Could you check a few things on this model? Use its own coordinates, in mm. A direction names the side the tool comes from. Coordinates: 2 decimals unless noted, no trailing zeros. Loops run counter-clockwise (first coordinate to the right, second up) from the corner with the lowest first, then second, coordinate; pieces in that order, holes last.
from build123d import *

# Parameters (mm, degrees)
EXTRUDE_1_DEPTH     = 20
CUT_EXTRUDE_1_DEPTH = 2


with BuildPart() as part:
    # 草圖1 → 填料-伸長1 (new body)
    with BuildSketch(Plane.XY):
        with BuildLine():
            Line((-63.421210963, 20), (-60, 20))
            Line((-60, 20), (-60, -20))
            Line((-60, -20), (-63.421210963, -20))
            ThreePointArc((-63.421210963, -20), (0, -66.5), (63.421210963, -20))
            Line((63.421210963, -20), (60, -20))
            Line((60, -20), (60, 20))
            Line((60, 20), (63.421210963, 20))
            ThreePointArc((63.421210963, 20), (0, 66.5), (-63.421210963, 20))
        make_face()
    extrude(amount=EXTRUDE_1_DEPTH)

    # 草圖2 → 除料-伸長1 (cut)
    with BuildSketch(Plane(origin=(0, 0, 0), x_dir=(-1, 0, 0), z_dir=(0, 0, -1))):
        with BuildLine():
            Line((-20, 63.421210963), (-20, -63.421210963))
            ThreePointArc((-20, -63.421210963), (0, -66.5), (20, -63.421210963))
            Line((20, -63.421210963), (20, 63.421210963))
            ThreePointArc((20, 63.421210963), (0, 66.5), (-20, 63.421210963))
        make_face()
    extrude(amount=-CUT_EXTRUDE_1_DEPTH, mode=Mode.SUBTRACT)


solid = part.part
(1) Imagine slicing it at A-A, the plane y = 8.5. Write out the boundary of the cut face in (x, z), and give its area (3 significant figures).
Answers:
outline: (-60, 0) - (-20, 0) - (-20, 2) - (20, 2) - (20, 0) - (60, 0) - (60, 20) - (-60, 20) - close
area: 2,320 mm2
(2) Imagine slicing it at C-C, the plane x = 29.5. Write out the boundary of the cut face in (y, z), and give its area (3 significant figures).
Answers:
outline: (-59.6, 0) - (59.6, 0) - (59.6, 20) - (-59.6, 20) - close
area: 2,380 mm2
(3) We'd pull the mould along Y, two halves only. Please class faces 1 (the face through (62, -20, 10)), 2 (the face through (-37, 1, 0)), 3 (the face through (-1.18, -66.49, 9.86)), 4 (the face through (60, 0, 10)): +Y half, -Y half, draft (parallel to the pull), parting line (faces both ways), or undercut.
Answers:
face 1: undercut
face 2: draft
face 3: -Y half
face 4: undercut
(4) Imagine slicing it at D-D, the plane x = 51.5. Write out the boundary of the cut face in (y, z), and give its area (3 significant figures).
Answers:
outline: (-42.07, 0) - (42.07, 0) - (42.07, 20) - (-42.07, 20) - close
area: 1,680 mm2
(5) I need wall thicknesses on probe 1 along Z at (x, y) = (-18, -40.5); probe 2 along X at (y, z) = (10, 19.25); probe 3 along X at (y, z) = (-47.5, 1). Which ranges of each line are inside material? Lowest first, please.
Answers:
probe 1: z = 2 to 20
probe 2: x = -60 to 60
probe 3: x = -46.54 to -20, 20 to 46.54
(6) Imagine slicing it at B-B, the plane z = 9. Write out the boundary of the cut face in (x, y), and give its area (3 significant figures).
Answers:
outline: (-63.42, -20) arc R66.5 ccw to (63.42, -20) - (60, -20) - (60, 20) - (63.42, 20) arc R66.5 ccw to (-63.42, 20) - (-60, 20) - (-60, -20) - close
area: 13,500 mm2
(7) Which directions (+Z, -Z, +X, -X, +Y, -Y) give clear straight access to the entire face, cutting with the end or side of a thin tool? Please do faces 5 (the face through (62, 20, 10)), 6 (the face through (37, 1, 0)), 7 (the face through (0, 1, 2)), 8 (the face through (-62, 20, 10)).
Answers:
face 5: +Z, -Z, +X
face 6: -Z, +X, -X, +Y, -Y
face 7: -Z, +Y, -Y
face 8: +Z, -Z, -X
(8) For pin 1 (12 mm diameter, centred on y = -35.5, z = 5.5, fed in from +X); pin 2 (1.7 mm diameter, centred on x = 61.5, z = 13, fed in from -Y); pin 3 (1 mm diameter, centred on x = -22.5, z = 17, fed in from +Y); pin 4 (6 mm diameter, centred on x = -30, y = 26.5, fed in from -Z), each with a flat end and sliding along its axis, tell me the tip position at first contact or that it passes through.
Answers:
pin 1: stops at x = 59.6
pin 2: stops at y = -27.27
pin 3: stops at y = 62.76
pin 4: stops at z = 0
